```python
from build123d import *

# Parameters (mm, degrees)
SKETCH1_R           = 11.295
BOSS_EXTRUDE1_DEPTH = 440
SKETCH4_R           = 6.5
CUT_EXTRUDE4_DEPTH  = 2
SKETCH5_R           = 7.5
CUT_EXTRUDE5_DEPTH  = 15
SKETCH6_R           = 6.5
CUT_EXTRUDE7_DEPTH  = 2
SKETCH8_R           = 7.5
CUT_EXTRUDE8_DEPTH  = 15


with BuildPart() as part:
    # Sketch1 → Boss-Extrude1 (new body)
    with BuildSketch(Plane.XY):
        Circle(SKETCH1_R)
    extrude(amount=BOSS_EXTRUDE1_DEPTH)

    # Sketch4 → Cut-Extrude4 (cut)
    with BuildSketch(Plane(origin=(0, 0, 0), x_dir=(-1, 0, 0), z_dir=(0, 0, -1))):
        Circle(SKETCH4_R)
    extrude(amount=-CUT_EXTRUDE4_DEPTH, mode=Mode.SUBTRACT)

    # Sketch5 → Cut-Extrude5 (cut)
    with BuildSketch(Plane(origin=(0, 0, 2), x_dir=(-1, 0, 0), z_dir=(0, 0, -1))):
        Circle(SKETCH5_R)
    extrude(amount=-CUT_EXTRUDE5_DEPTH, mode=Mode.SUBTRACT)

    # Sketch6 → Cut-Extrude7 (cut)
    with BuildSketch(Plane.XY.offset(440)):
        Circle(SKETCH6_R)
    extrude(amount=-CUT_EXTRUDE7_DEPTH, mode=Mode.SUBTRACT)

    # Sketch8 → Cut-Extrude8 (cut)
    with BuildSketch(Plane.XY.offset(438)):
        Circle(SKETCH8_R)
    extrude(amount=-CUT_EXTRUDE8_DEPTH, mode=Mode.SUBTRACT)


solid = part.part
```
Model file for the job. Use its own axes, mm. A direction names the side the tool comes from. Coordinates: 2 decimals unless noted, no trailing zeros. Write each loop counter-clockwise with the first axis right and the second up, starting at its lowest first coordinate (ties: lowest second). Pieces come first, ordered by that corner, then holes. Notation, with made-up numbers: (-32, 36) - (16, 36) arc R21 cw to (16, 43) - close; hole circle Ø10 at (-7.75, -18). An arc over 180 degrees is marked (long way). One line per question, with ' | ' between items. Start each with the question number.
Q1. Pin check, flat tips, straight feed: pin 1 (2 mm diameter, centred on x = -2.5, z = 393, fed in from +Y); pin 2 (8 mm diameter, centred on x = -7.5, z = 222, fed in from -Y); pin 3 (10 mm diameter, centred on x = -8, z = 140.5, fed in from -Y). Stop position of each tip, or through.
Q2. Cut at A-A, the plane y = 0. List the corners of the cut face in (x, z) (3 decimals), then the cut area to 3 significant figures.
Q3. 3-axis set-ups, long thin cutter, end or side, ignore diameter. For faces 1 (the face through (-5.158, -3.955, 439.014)), 2 (the face through (0, 0, 17)), 3 (the face through (-2.449, -11.026, 216.92)): which of +Z, -Z, +X, -X, +Y, -Y reach the whole face in a straight line?
Q4. Pull direction Z, two halves, no side cores. Call faces 4 (the face through (7.493, 0.33, 9.395)), 5 (the face through (5.158, -3.955, 0.986)), 6 (the face through (5, -5, 0)), 7 (the face through (5, -5, 440)): pulls with the +Z half, pulls with the -Z half, needs draft (parallel to the pull), parting line crosses it, or undercut.
Q5. Drill centre lines: line 1 (Z direction, x = -7, y = 0.75); line 2 (Y direction, x = 0, z = 0.6) (3 decimals); line 3 (Y direction, x = 0, z = 12.25) (3 decimals). Where is each one in solid material? Low to high. Write a range as [from, to].
Q6. Cut at C-C, the plane z = 354. List the corners of the cut face in (x, y) (3 decimals), then the cut area to 3 significant figures.
Answer below:
1) pin 1: y = 11.19 | pin 2: y = -10.74 | pin 3: y = -10.89
2) outline: (-11.295, 0) - (-6.5, 0) - (-6.5, 2) - (-7.5, 2) - (-7.5, 17) - (7.5, 17) - (7.5, 2) - (6.5, 2) - (6.5, 0) - (11.295, 0) - (11.295, 440) - (6.5, 440) - (6.5, 438) - (7.5, 438) - (7.5, 423) - (-7.5, 423) - (-7.5, 438) - (-6.5, 438) - (-6.5, 440) - (-11.295, 440) - close | area: 9,440 mm^2
3) face 1: +Z | face 2: none | face 3: +Z, -Z
4) face 4: undercut | face 5: needs draft | face 6: pulls with the -Z half | face 7: pulls with the +Z half
5) line 1: [0, 2], [17, 423], [438, 440] | line 2: [-11.295, -6.5], [6.5, 11.295] | line 3: [-11.295, -7.5], [7.5, 11.295]
6) outline: circle Ø22.59 at (0, 0) | area: 401 mm^2
